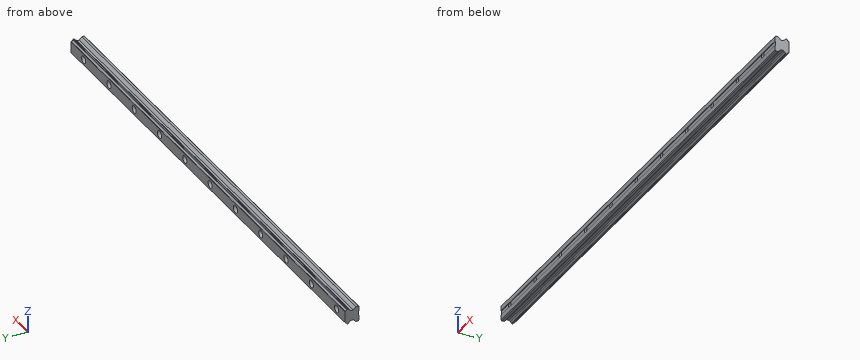
from build123d import *

# Parameters (mm, degrees)
BOSS_EXTRUDE1_DEPTH = 650
LPATTERN1_COUNT     = 9
LPATTERN1_PITCH     = 60


with BuildPart() as part:
    # Sketch1 → Boss-Extrude1 (new body)
    with BuildSketch(Plane(origin=(-20, 0, 0), x_dir=(0, 0, -1), z_dir=(1, 0, 0))):
        with BuildLine():
            Line((-10, 4.000077248), (-10, 1))
            Line((-10, 1), (-9, 0))
            Line((-9, 0), (-3, 0))
            Line((-3, 0), (-2.5, 0.5))
            Line((-2.5, 0.5), (2.5, 0.5))
            Line((2.5, 0.5), (3, 0))
            Line((3, 0), (9, 0))
            Line((9, 0), (10, 1))
            Line((10, 1), (10, 4.000077248))
            Line((10, 4.000077248), (6.550048828, 7.449951172))
            Line((6.550048828, 7.449951172), (6.550048828, 10.379235268))
            Line((6.550048828, 10.379235268), (7.765945541, 11.595131504))
            ThreePointArc((7.765945541, 11.595131504), (8.344873878, 12.735447983), (9.485190198, 13.314376637))
            Line((9.485190198, 13.314376637), (10, 13.82918644))
            Line((10, 13.82918644), (10, 15.160037041))
            Line((10, 15.160037041), (9.472673258, 15.687363783))
            ThreePointArc((9.472673258, 15.687363783), (8.344874488, 16.264307267), (7.767930373, 17.392105714))
            Line((7.767930373, 17.392105714), (7.160036564, 18))
            Line((7.160036564, 18), (-7.160036564, 18))
            Line((-7.160036564, 18), (-7.767930373, 17.392105714))
            ThreePointArc((-7.767930373, 17.392105714), (-8.344874488, 16.264307267), (-9.472673258, 15.687363783))
            Line((-9.472673258, 15.687363783), (-10, 15.160037041))
            Line((-10, 15.160037041), (-10, 13.82918644))
            Line((-10, 13.82918644), (-9.485190198, 13.314376637))
            ThreePointArc((-9.485190198, 13.314376637), (-8.344873878, 12.735447983), (-7.765945541, 11.595131504))
            Line((-7.765945541, 11.595131504), (-6.550048828, 10.379235268))
            Line((-6.550048828, 10.379235268), (-6.550048828, 7.449951172))
            Line((-6.550048828, 7.449951172), (-10, 4.000077248))
        make_face()
    extrude(amount=BOSS_EXTRUDE1_DEPTH)

    # Sketch2 → Cut-Revolve1 (revolve, cut)
    with BuildSketch(Plane.XY):
        Polygon((0, 18), (4.75, 18), (4.75, 9.5), (3, 9.5), (3, 0), (0, 0), align=None)
    revolve(axis=Axis((0, 0, 0), (0, 1, 0)), mode=Mode.SUBTRACT)

    # Sketch3 → Cut-Revolve2 (revolve, cut)
    with BuildSketch(Plane.XY):
        Polygon((60, 18), (64.75, 18), (64.75, 9.5), (63, 9.5), (63, 0), (60, 0), align=None)
    revolve(axis=Axis((60, 0, 0), (0, 1, 0)), mode=Mode.SUBTRACT)

    # Sketch4 → Cut-Revolve3 (revolve, cut)
    with BuildSketch(Plane.XY):
        Polygon((120, 18), (124.75, 18), (124.75, 9.5), (123, 9.5), (123, 0), (120, 0), align=None)
    cut_revolve3 = revolve(axis=Axis((120, 0, 0), (0, 1, 0)), mode=Mode.SUBTRACT)

    # LPattern1: Cut-Revolve3 ×9
    with Locations(*[(i * LPATTERN1_PITCH, 0, 0) for i in range(1, LPATTERN1_COUNT)]):
        add(cut_revolve3, mode=Mode.SUBTRACT)


solid = part.part
Verification items for the finished model (mm, model axes). Coordinates: 2 decimals unless noted, no trailing zeros. Order: outer loops, then holes, each group sorted by start corner. A loop starts at its lowest first (then second) coordinate and runs counter-clockwise, first axis right, second up.
Item 1: Depth check by flat-ended pin: pin 1 (5.5 mm diameter, centred on x = 180, z = 0, fed in from -Y); pin 2 (8 mm diameter, centred on x = 360, z = 0, fed in from +Y); pin 3 (5.5 mm diameter, centred on x = 446.5, z = 0, fed in from -Y); pin 4 (0.9 mm diameter, centred on x = 323.5, y = 8.5, fed in from +Z). Enter the tip coordinate at first touch or a pass-through.
Filled in:
pin 1: passes through
pin 2: stops at y = 9.5
pin 3: stops at y = 0.25
pin 4: stops at z = 6.55
Item 2: Section check A-A, the plane x = 405.5. Enter the section's corners in (y, z).
Filled in:
outline: (0, -9) - (1, -10) - (4, -10) - (7.45, -6.55) - (10.38, -6.55) - (11.6, -7.77) arc R2.06 cw to (13.31, -9.49) - (13.83, -10) - (15.16, -10) - (15.69, -9.47) arc R2.06 cw to (17.39, -7.77) - (18, -7.16) - (18, 7.16) - (17.39, 7.77) arc R2.06 cw to (15.69, 9.47) - (15.16, 10) - (13.83, 10) - (13.31, 9.49) arc R2.06 cw to (11.6, 7.77) - (10.38, 6.55) - (7.45, 6.55) - (4, 10) - (1, 10) - (0, 9) - (0, 3) - (0.5, 2.5) - (0.5, -2.5) - (0, -3) - close
Item 3: Material ranges on L1, parallel to Z at x = 120, y = 7.5; L2, parallel to Z at x = 540, y = 11.5; L3, parallel to Z at x = 149.5, y = 17, recorded low to high.
Filled in:
L1: z = -6.55 to -3, 3 to 6.55
L2: z = -7.67 to -4.75, 4.75 to 7.67
L3: z = -7.87 to 7.87
